```python
from build123d import *

# Parameters (mm, degrees)
SKETCH1_W                  = 292.1
SKETCH1_H                  = 76.2
BOSS_EXTRUDE1_DEPTH        = 4.7625
SKETCH2_R                  = 32.258
CUT_EXTRUDE1_DEPTH         = 10.525
FILLET1_R                  = 34.925
F_10_32_TAPPED_HOLE2_D     = 4.0386
F_10_32_TAPPED_HOLE2_DEPTH = 19.05
F_10_32_TAPPED_HOLE2_TIP   = 1.213317848


with BuildPart() as part:
    # Sketch1 → Boss-Extrude1 (new body, symmetric)
    with BuildSketch(Plane.XY):
        Rectangle(SKETCH1_W, SKETCH1_H)
    extrude(amount=BOSS_EXTRUDE1_DEPTH, both=True)

    # Sketch2 → Cut-Extrude1 (cut, through all)
    with BuildSketch(Plane.XY.offset(4.7625)):
        with Locations((-107.95, 0)):
            Circle(SKETCH2_R)
        with Locations((-35.983333333, 0)):
            Circle(SKETCH2_R)
        with Locations((35.983333333, 0)):
            Circle(SKETCH2_R)
        with Locations((107.95, 0)):
            Circle(SKETCH2_R)
    extrude(amount=-CUT_EXTRUDE1_DEPTH, mode=Mode.SUBTRACT)

    # Fillet1
    fillet1_edges = [part.edges().sort_by_distance(p)[0] for p in [
        (-146.05, 38.1, 0),
        (146.05, 38.1, 0),
        (146.05, -38.1, 0),
        (-146.05, -38.1, 0),
    ]]
    fillet(fillet1_edges, radius=FILLET1_R)

    # #10-32 Tapped Hole2
    with Locations(Plane(origin=(0, 38.1, 0), x_dir=(1, 0, 0), z_dir=(0, 1, 0))):
        with Locations((-78.105, 0), (78.105, 0)):
            Hole(F_10_32_TAPPED_HOLE2_D / 2, depth=F_10_32_TAPPED_HOLE2_DEPTH)
            with Locations((0, 0, -(F_10_32_TAPPED_HOLE2_DEPTH + F_10_32_TAPPED_HOLE2_TIP / 2))):  # 118° drill point
                Cone(0, F_10_32_TAPPED_HOLE2_D / 2, F_10_32_TAPPED_HOLE2_TIP, mode=Mode.SUBTRACT)


solid = part.part
```
The model under review builds one solid part; all positions refer to its coordinate system, in mm. Round coordinates to 2 decimals unless told otherwise and drop trailing zeros. Order: outer loops, then holes, each group sorted by start corner. A loop starts at its lowest first (then second) coordinate and runs counter-clockwise, first axis right, second up. Notation, with made-up numbers: (11, 20.5) -> (59, 20.5) arc R15 cw to (59, 25.5) -> close; hole circle Ø9 at (86, 7). An arc over 180 degrees is marked (long way). Use a Markdown table: item, result.
Q1. Clearance check with flat-ended pins moving along their axes: P1, Ø5, axis at y = -7, z = 0.5, coming from the +X side; P2, Ø4, axis at y = 18.5, z = -2.5, coming from the -X side. State where each tip first meets the part, or that it passes through.
Values:
| item | result |
|---|---|
| P1 | stops at x = 146.02 |
| P2 | stops at x = -143.41 |
Q2. We need section C-C on x = -7.5. Write out the cut boundary in (y, z), then the cut area to 3 significant figures.
Values:
| item | result |
|---|---|
| outline | (-38.1, -4.76) -> (-15.14, -4.76) -> (-15.14, 4.76) -> (-38.1, 4.76) -> close; (15.14, -4.76) -> (38.1, -4.76) -> (38.1, 4.76) -> (15.14, 4.76) -> close |
| area | 437 mm^2 |
Q3. We need section A-A on y = 0. Write out the cut boundary in (x, z), then the cut area to 3 significant figures.
Values:
| item | result |
|---|---|
| outline | (-146.05, -4.76) -> (-140.21, -4.76) -> (-140.21, 4.76) -> (-146.05, 4.76) -> close; (-75.69, -4.76) -> (-68.24, -4.76) -> (-68.24, 4.76) -> (-75.69, 4.76) -> close; (-3.73, -4.76) -> (3.73, -4.76) -> (3.73, 4.76) -> (-3.73, 4.76) -> close; (68.24, -4.76) -> (75.69, -4.76) -> (75.69, 4.76) -> (68.24, 4.76) -> close; (140.21, -4.76) -> (146.05, -4.76) -> (146.05, 4.76) -> (140.21, 4.76) -> close |
| area | 324 mm^2 |
Q4. For line 1 (X direction, y = 17, z = 0); line 2 (Y direction, x = 107.95, z = 1.25); line 3 (X direction, y = 2.5, z = 2.75), list the stretches that pass through material, from the lowest coordinate up.
Values:
| item | result |
|---|---|
| line 1 | x = -143.2 to -135.36, -80.54 to -63.4, -8.57 to 8.57, 63.4 to 80.54, 135.36 to 143.2 |
| line 2 | y = -38.1 to -32.26, 32.26 to 38.1 |
| line 3 | x = -146.05 to -140.11, -75.79 to -68.14, -3.82 to 3.82, 68.14 to 75.79, 140.11 to 146.05 |
Q5. Mouldability with a two-part tool opening along X and no side actions: class faces 1 (the flat face through (-2, -38.1, 0)), 2 (the flat face through (-146.05, 0, 0)), 3 (the cylindrical face through (3.757, 1.418, 0.067)) as +X half, -X half, draft (parallel to the pull), parting line (faces both ways), or undercut.
Values:
| item | result |
|---|---|
| face 1 | draft |
| face 2 | -X half |
| face 3 | undercut |
Q6. We need section B-B on x = 90. Write out the cut boundary in (y, z).
Values:
| item | result |
|---|---|
| outline | (-38.1, -4.76) -> (-26.8, -4.76) -> (-26.8, 4.76) -> (-38.1, 4.76) -> close; (26.8, -4.76) -> (38.1, -4.76) -> (38.1, 4.76) -> (26.8, 4.76) -> close |
Q7. We need section D-D on y = -20.5. Write out the cut boundary in (x, z).
Values:
| item | result |
|---|---|
| outline | (-141.45, -4.76) -> (-132.86, -4.76) -> (-132.86, 4.76) -> (-141.45, 4.76) -> close; (-83.04, -4.76) -> (-60.89, -4.76) -> (-60.89, 4.76) -> (-83.04, 4.76) -> close; (-11.08, -4.76) -> (11.08, -4.76) -> (11.08, 4.76) -> (-11.08, 4.76) -> close; (60.89, -4.76) -> (83.04, -4.76) -> (83.04, 4.76) -> (60.89, 4.76) -> close; (132.86, -4.76) -> (141.45, -4.76) -> (141.45, 4.76) -> (132.86, 4.76) -> close |
